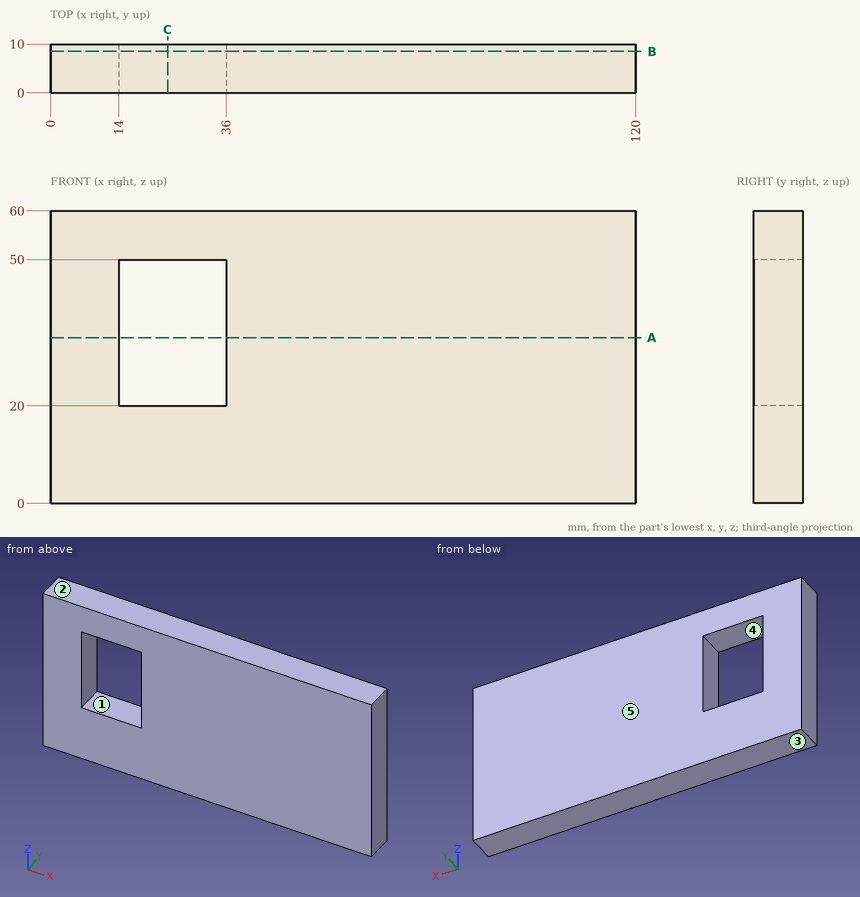
Design review of the part shown in the three views and the two pictorial views. Dimensions are in mm from the part's minimum x, y and z. A direction names the side the tool comes from. Coordinates: 2 decimals unless noted, no trailing zeros. Loops run counter-clockwise (first coordinate to the right, second up) from the corner with the lowest first, then second, coordinate; pieces in that order, holes last.
(1) Tool access review of the marked faces 4 and 5: name each direction out of +Z, -Z, +X, -X, +Y, -Y from which nothing blocks a thin tool from reaching the whole face with its end or side.
Determined:
face 4: +Y, -Y
face 5: +Z, -Z, +X, -X, +Y
(2) Consider section C-C, the plane x = 24. Give the boundary of the cut face in (y, z).
Determined:
outline: (0, 0) - (10, 0) - (10, 20) - (0, 20) - close; (0, 50) - (10, 50) - (10, 60) - (0, 60) - close
(3) Consider section B-B, the plane y = 8.5. Give the boundary of the cut face in (x, z), plus the area to 3 significant figures.
Determined:
outline: (0, 0) - (120, 0) - (120, 60) - (0, 60) - close; hole (14, 20) - (36, 20) - (36, 50) - (14, 50) - close
area: 6,540 mm2
(4) Consider section A-A, the plane z = 34. Give the boundary of the cut face in (x, y), plus the area to 3 significant figures.
Determined:
outline: (0, 0) - (14, 0) - (14, 10) - (0, 10) - close; (36, 0) - (120, 0) - (120, 10) - (36, 10) - close
area: 980 mm2
(5) Wall thickness on L1, parallel to X at y = 6.5, z = 39.5; L2, parallel to Z at x = 30, y = 6.75: over which ranges is each line inside the solid? List them lowest first.
Determined:
L1: x = 0 to 14, 36 to 120
L2: z = 0 to 20, 50 to 60
(6) Draft analysis for pull direction Z (two halves, no side actions). For the marked faces 1, 2 and 3, state which applies: +Z half, -Z half, draft (parallel to the pull), parting line (faces both ways), or undercut.
Determined:
face 1: undercut
face 2: +Z half
face 3: -Z half
